Source: CAD feature listing. Evaluate the final solid. Frame: model axes, mm. A direction names the side the tool comes from. Give positions to 0.01 mm unless a question says otherwise; leave off trailing zeros. Loops run counter-clockwise (first coordinate to the right, second up) from the corner with the lowest first, then second, coordinate; pieces in that order, holes last. Notation, with made-up numbers: M -8,53.25 L 17,53.25 A20 cw 17,62.25 Z; hole C 83.5,-6 d5. An arc over 180 degrees is marked long. Write item = value, one per line.
from build123d import *

# Parameters (mm, degrees)
SKETCH1_R           = 34.925
SKETCH1_R_2         = 25.4
BOSS_EXTRUDE1_DEPTH = 18.796


with BuildPart() as part:
    # Sketch1 → Boss-Extrude1 (new body)
    with BuildSketch(Plane.XY):
        Circle(SKETCH1_R)
        Circle(SKETCH1_R_2, mode=Mode.SUBTRACT)
    extrude(amount=BOSS_EXTRUDE1_DEPTH)

    # Cut-Sweep1: sweep along a path in groove path
    with BuildLine(Plane.XY.offset(11.0109)) as cut_sweep1_path:
        CenterArc((0, 0), 34.925, 0, 360)
    # groove → Cut-Sweep1 (sweep, cut)
    with BuildSketch(Plane(origin=(0, 0, 0), x_dir=(0, 0, -1), z_dir=(1, 0, 0))):
        Polygon((-15.7734, 34.987595096), (-15.7734, 32.193595096), (-11.0109, 32.193595096), (-10.9982, 34.987595096), (-7.8232, 34.987595096), (-7.8232, 32.193595096), (-3.048, 32.193595096), (-3.048, 34.987595096), (-3.048, 38.125839406), (-15.7734, 38.125839406), align=None)
    sweep(path=cut_sweep1_path.line, mode=Mode.SUBTRACT)


solid = part.part
1. First-contact query: pin 1 Ø6 at (y, z) = (-20, 14.5) entering from -X; pin 2 Ø5 at (y, z) = (26, 11.5) entering from +X; pin 3 Ø8 at (y, z) = (26.5, 11.5) entering from +X. Flat tips, straight axial feed; report the tip coordinate or a pass-through.
Derived:
pin_1 = -30.35
pin_2 = 25.79
pin_3 = 26.68
2. Reachability of faces 4 (the cylindrical face through (30.707, 9.67, 5.402)), 5 (the cylindrical face through (-27.715, -21.251, 17.264)) from +Z, -Z, +X, -X, +Y, -Y: full face, straight path, thin tool, end or side. Return the list, or none.
Derived:
face_4 = none
face_5 = +Z, -Z
3. Pull-direction query (X, two-part tool) for faces 1 (the flat face through (2, -26, 0)), 2 (the cylindrical face through (-27.715, -21.251, 1.503)), 3 (the cylindrical face through (-5.506, -24.796, 9.266)); classes: +X half, -X half, draft (parallel to the pull), parting line (faces both ways), or undercut.
Derived:
face_1 = draft
face_2 = parting line
face_3 = undercut
4. Material intervals for probe 1 along Z at (x, y) = (-31.5, -8); probe 2 along Y at (x, z) = (0, 4.75); probe 3 along X at (y, z) = (17, 13), sorted ascending. Write a range as from..to.
Derived:
probe_1 = 0..3.05, 7.82..11.01, 15.77..18.8
probe_2 = -32.19..-25.4, 25.4..32.19
probe_3 = -27.34..-18.87, 18.87..27.34
5. Cut plane A-A, the plane z = 14. Return the cut outline in (x, y), then the cut area to 3 significant figures.
Derived:
outline = C 0,0 d64.39; hole C 0,0 d50.8
area = 1,230 mm²
